```python
from build123d import *

# Parameters (mm, degrees)
BOSS_EXTRUDE3_DEPTH = 1000


with BuildPart() as part:
    # Sketch1 → Boss-Extrude3 (new body)
    with BuildSketch(Plane(origin=(0, 0, -500), x_dir=(0, 0, -1), z_dir=(1, 0, 0))):
        Polygon((-642.779409885, 256.120502949), (-644.914388657, 255.904585123), (-646.200299263, 255.71128726), (-646.685421467, 255.589991808), (-647.101521492, 255.439013243), (-647.425472736, 255.27459383), (-647.714614868, 255.077391863), (-647.978484631, 254.839211702), (-648.275375366, 254.489988089), (-648.636221886, 253.934204578), (-649.123728275, 252.929896116), (-649.30999279, 252.462893724), (-649.766325951, 250.954300165), (-650.021493435, 249.423295259), (-650.094270706, 247.779801488), (-650.038719177, 246.605500579), (-649.602711201, 243.699401617), (-648.441672325, 239.474505186), (-647.353470325, 236.322000623), (-645.422577858, 231.728598475), (-643.051326275, 227.357104421), (-640.120506287, 222.93870151), (-636.568427086, 218.405202031), (-632.264912128, 213.678896427), (-627.326071262, 208.981901407), (-621.761500835, 204.359397292), (-615.521609783, 199.795395136), (-608.5485816, 195.271506906), (-600.728929043, 190.76859951), (-596.005380154, 188.305199146), (-587.184429169, 184.160396457), (-577.917218208, 180.371597409), (-568.137705326, 176.927000284), (-557.888925076, 173.8602072), (-547.180473804, 171.18909955), (-536.01872921, 168.915003538), (-534.444212914, 168.630793691), (-521.650195122, 166.604802012), (-508.135974407, 164.908796549), (-492.430597544, 163.390293717), (-475.852102041, 162.333399057), (-459.896713495, 161.8847996), (-444.510787725, 162.004098296), (-429.100692272, 162.644594908), (-413.232386112, 163.816794753), (-396.332412958, 165.601596236), (-379.418700933, 167.905002832), (-361.880987883, 170.800805092), (-343.654692173, 174.315303564), (-324.638485909, 178.4837991), (-304.697185755, 183.361396194), (-286.849200726, 188.203394413), (-270.105808973, 193.222895265), (-252.515107393, 199.067205191), (-235.948398709, 205.165296793), (-219.85130012, 211.677998304), (-204.168900847, 218.616306782), (-191.308796406, 224.782302976), (-180.752694607, 230.286598206), (-173.555895686, 234.368100762), (-168.321296573, 237.659201026), (-163.910001516, 240.874201059), (-160.164996982, 244.140699506), (-156.561002135, 247.982501984), (-153.336599469, 252.174496651), (-150.913998485, 255.951285362), (-156.019702554, 250.904113054), (-161.501795053, 246.226206422), (-167.419299483, 241.865903139), (-173.723697662, 237.868800759), (-180.422201753, 234.187602997), (-187.979504466, 230.538204312), (-198.573499918, 226.002797484), (-216.145798564, 219.094693661), (-228.632703424, 214.508801699), (-240.639105439, 210.572898388), (-252.248704433, 207.256004214), (-264.682114124, 204.265296459), (-276.933789253, 201.882794499), (-289.279103279, 200.03400743), (-301.696509123, 198.68889451), (-314.927399158, 197.707295418), (-329.930603504, 197.033897042), (-346.439599991, 196.817696095), (-362.657696009, 197.159305215), (-378.566503525, 198.04109633), (-394.465506077, 199.431404471), (-396.365493536, 199.629202485), (-413.707196712, 201.723203063), (-431.453704834, 204.358592629), (-450.356990099, 207.704395056), (-468.465685844, 211.488306522), (-485.652685165, 215.641096234), (-502.897024155, 220.307901502), (-521.483182907, 225.811600685), (-541.911184788, 232.310399413), (-564.286708832, 239.661693573), (-582.044124603, 245.254397392), (-595.689117908, 249.179899693), (-606.637179852, 251.971691847), (-616.060674191, 253.978610039), (-624.257326126, 255.313187838), (-631.537616253, 256.076693535), (-637.538611889, 256.317704916), align=None)
    extrude(amount=BOSS_EXTRUDE3_DEPTH)


solid = part.part
```
For this review, take the finished solid that the model builds, in its own axes (mm). A direction names the side the tool comes from. Give positions to 0.01 mm unless a question says otherwise; leave off trailing zeros.
1) For faces 1 (the face through (493, 209.57, -40.72)), 2 (the face through (493, 176.37, -165.72)), list the 3-axis set-ups (+Z, -Z, +X, -X, +Y, -Y) from which the entire face can be reached by the end or side of a thin tool; tool diameter is ignored.
2) The part is to be moulded in two halves that separate along Z. For faces 3 (the face through (1000, 199, -41)), 4 (the face through (493, 164.697, -95.099)), 5 (the face through (493, 222.597, -292.763)), say which applies: released by +Z, released by -Z, zero draft, split by the parting line, or undercut.
3) Insertion check: pin 1 (2 mm diameter, centred on x = 211, y = 214, fed in from -Z); pin 2 (12 mm diameter, centred on x = 673, y = 217.5, fed in from -Z); pin 3 (4 mm diameter, centred on x = 776, y = 211.5, fed in from -Z). Each pin has a flat end and moves straight along its axis. Give the tip position at first contact, or say it passes through.
4) Wall thickness on line 1 (Y direction, x = 185.5, z = -44.5); line 2 (Y direction, x = 343, z = -65): over which ranges is each line inside the solid? List them lowest first.
Derived:
1. face 1: +X, -X, +Y
1. face 2: -Z, +X, -X, -Y
2. face 3: zero draft
2. face 4: released by -Z
2. face 5: undercut
3. pin 1: stops at z = -287.66
3. pin 2: stops at z = -306.02
3. pin 3: stops at z = -284.27
4. line 1: y = 161.92 to 208.78
4. line 2: y = 162.4 to 204.99
